Geometry check sheet. Reference: the model listing, model coordinates, mm. A direction names the side the tool comes from. Give positions to 0.01 mm unless a question says otherwise; leave off trailing zeros. Write each loop counter-clockwise with the first axis right and the second up, starting at its lowest first coordinate (ties: lowest second). Pieces come first, ordered by that corner, then holes.
(1) Cross-section at A-A (y = -5.5). Record the boundary of the cut face in (x, z), and give its area (3 significant figures).
(2) Mould release check, pull along X, two halves, no side actions. Record for faces 1 (the flat face through (-5, 0, 6)), 2 (the cylindrical face through (-4.3, -12.52, 68.72)), 3 (the flat face through (37, -13, -9.976)): +X half, -X half, draft (parallel to the pull), parting line (faces both ways), or undercut.
(3) Tool access check on faces 4 (the flat face through (-5, -25.4, 6)), 5 (the flat face through (-26.636, -13, 24)). Record the directions out of +Z, -Z, +X, -X, +Y, -Y that give a thin tool (end or side, any length) a straight path to the whole face; none if there is none.
(4) Cross-section at B-B (x = -25). Record the boundary of the cut face in (y, z), and give its area (3 significant figures).
(5) Cross-section at C-C (z = 5.5). Record the boundary of the cut face in (x, y).
(6) Depth check by flat-ended pin: P1, Ø6, axis at y = -9, z = 16.5, coming from the -X side; P2, Ø1.5, axis at x = 48, y = -15.5, coming from the +Z side; P3, Ø12, axis at y = -8, z = 39, coming from the +X side. Enter the tip coordinate at first touch or a pass-through.
(7) Thickness scan on line 1 along X through (y, z) = (-6, 41); line 2 along X through (y, z) = (-9, -13); line 3 along Z through (x, y) = (-34.5, -18.5). Record the ranges inside material, lowest first.
```python
from build123d import *

# Parameters (mm, degrees)
F1_DEPTH = 25.4


with BuildPart() as f1:
    # F0 (on Front) → F1 (new body)
    with BuildSketch(Plane.XZ):
        with BuildLine():
            Line((-26.635719, 56.048136), (-26.635719, -9.358496))
            Line((-26.635719, -9.358496), (-59.750397, -9.358496))
            Line((-59.750397, -9.358496), (-66.126518, -9.358496))
            ThreePointArc((-66.126518, -9.358496), (-78.981595, -22.213573), (-66.126518, -35.06865))
            Line((-66.126518, -35.06865), (57.282224, -33.21752))
            ThreePointArc((57.282224, -33.21752), (71.156125, -21.220004), (56.665178, -9.97554))
            Line((56.665178, -9.97554), (17.174384, -9.97554))
            Line((17.174384, -9.97554), (17.174384, 55.842455))
            ThreePointArc((17.174384, 55.842455), (-4.670679, 68.722974), (-26.635719, 56.048136))
        make_face()
    extrude(amount=F1_DEPTH)


solid = f1.part
```
Reply:
1. outline: (-66.13, -35.07) - (57.28, -33.22) arc R11.86 ccw (long way) to (56.67, -9.98) - (17.17, -9.98) - (17.17, 55.84) arc R25.17 ccw to (-26.64, 56.05) - (-26.64, -9.36) - (-66.13, -9.36) arc R12.86 ccw to start
1. area: 6,820 mm2
2. face 1: draft
2. face 2: parting line
2. face 3: undercut
3. face 4: +Z, -Z, +X, -X, -Y
3. face 5: +Z, -X, +Y, -Y
4. outline: (-25.4, -34.45) - (0, -34.45) - (0, 58.55) - (-25.4, 58.55) - close
4. area: 2,360 mm2
5. outline: (-26.64, -25.4) - (17.17, -25.4) - (17.17, 0) - (-26.64, 0) - close
6. P1: stops at x = -26.64
6. P2: stops at z = -9.98
6. P3: stops at x = 17.17
7. line 1: x = -26.64 to 17.17
7. line 2: x = -75.09 to 67.53
7. line 3: z = -34.59 to -9.36
